Could you check a few things on this model? Use its own coordinates, in mm. Face numbers are marked on the shaded views. A direction names the side the tool comes from. Give positions to 0.01 mm unless a question says otherwise; leave off trailing zeros. Order: outer loops, then holes, each group sorted by start corner. A loop starts at its lowest first (then second) coordinate and runs counter-clockwise, first axis right, second up. Notation, with made-up numbers: M 32.25,77.25 L 48.25,77.25 A24 ccw 48.25,94.25 Z; hole C 44.25,-18.5 d10. An arc over 180 degrees is marked long. Return JSON: item names as keys, results as strings. Group by question number.
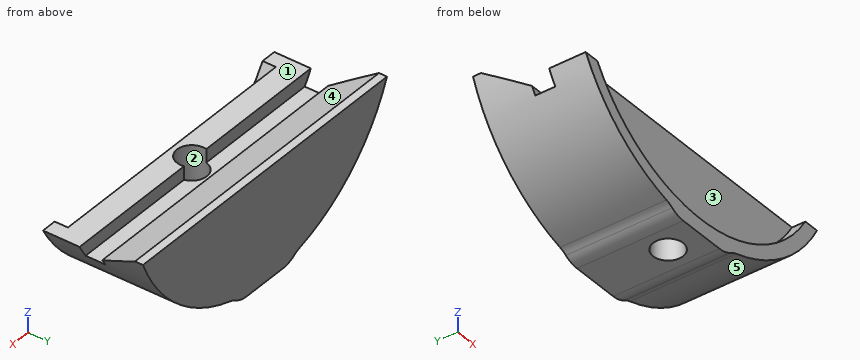
```python
from build123d import *

# Parameters (mm, degrees)
SKETCH_1_R                  = 26
EXTRUDE_1_DEPTH             = 14
CUT_EXTRUDE_1_DEPTH         = 30
HOLE_WIZARD_M32_D           = 3.4
HOLE_WIZARD_M32_CBORE_D     = 6.6
HOLE_WIZARD_M32_CBORE_DEPTH = 3
EXTRUDE_START               = 2
SKETCH_12_R                 = 26
SKETCH_12_R_2               = 24
EXTRUDE_2_DEPTH             = 2
CUT_EXTRUDE_START           = -8
CUT_EXTRUDE_4_DEPTH         = 8
FILLET_2_R                  = 1
SKETCH_18_R                 = 6
CUT_EXTRUDE_5_DEPTH         = 3
CUT_EXTRUDE_START_2         = -10
CUT_EXTRUDE_6_DEPTH         = 10
M4X0_71_D                   = 3.3
M4X0_71_DEPTH               = 11.5
M4X0_71_TIP                 = 0.991420021
SKETCH_20_W                 = 50.531548996
SKETCH_20_H                 = 7
CUT_EXTRUDE_7_DEPTH         = 2
SKETCH_24_W                 = 22.63069338
SKETCH_24_H                 = 1
EXTRUDE_3_DEPTH             = 2
SKETCH_25_W                 = 27.749072331
SKETCH_25_H                 = 11.312162615
CUT_EXTRUDE_8_DEPTH         = 60.799665638
SKETCH_26_W                 = 2
SKETCH_26_H                 = 3
CUT_EXTRUDE_10_DEPTH        = 59.164737265
EXTRUDE_START_2             = -16
EXTRUDE_5_DEPTH             = 16
FILLET_3_R                  = 4
FILLET_4_R                  = 4
HOLE_WIZARD_M41_D           = 4.5


with BuildPart() as part:
    # Эскиз1 → Бобышка-Вытянуть1 (new body)
    with BuildSketch(Plane(origin=(0, 0, 0), x_dir=(1, 0, 0), z_dir=(0, 1, 0))):
        with Locations(Location((0, 0, 0), (0, 0, 270))):
            Circle(SKETCH_1_R)
    extrude(amount=EXTRUDE_1_DEPTH)

    # Эскиз2 → Вырез-Вытянуть1 (cut, symmetric)
    with BuildSketch(Plane(origin=(0, 0, 0), x_dir=(0, 0, -1), z_dir=(1, 0, 0))):
        Polygon((13.654700538, 6), (-13.654700538, 6), (-9.728718708, 12.8), (-9.728718708, 14), (9.728718708, 14), (9.728718708, 12.8), align=None)
    extrude(amount=CUT_EXTRUDE_1_DEPTH, both=True, mode=Mode.SUBTRACT)

    # Цековка для винта с внутренним шестигранником M32 (through all)
    with Locations(Plane(origin=(0, 6, 0), x_dir=(1, 0, 0), z_dir=(0, 1, 0))):
        with Locations((-12.5, 0), (12.5, 0), (-6, 0), (6, 0)):
            CounterBoreHole(HOLE_WIZARD_M32_D / 2, HOLE_WIZARD_M32_CBORE_D / 2, HOLE_WIZARD_M32_CBORE_DEPTH)

    # Эскиз12 → Бобышка-Вытянуть2 (add)
    with BuildSketch(Plane.XZ.offset(EXTRUDE_START)):
        with Locations(Location((0, 0, 0), (0, 0, 270))):
            Circle(SKETCH_12_R)
        with Locations(Location((0, 0, 0), (0, 0, 270))):
            Circle(SKETCH_12_R_2, mode=Mode.SUBTRACT)
    extrude(amount=-EXTRUDE_2_DEPTH)

    # Эскиз17 → Вырез-Вытянуть4 (cut)
    with BuildSketch(Plane(origin=(0, 14, 0), x_dir=(1, 0, 0), z_dir=(0, 1, 0)).offset(CUT_EXTRUDE_START)):
        with BuildLine():
            Line((-24.111242861, -9.728718708), (24.111242861, -9.728718708))
            ThreePointArc((24.111242861, -9.728718708), (0, -26), (-24.111242861, -9.728718708))
        make_face()
    extrude(amount=CUT_EXTRUDE_4_DEPTH, mode=Mode.SUBTRACT)

    # Скругление2
    fillet_2_edges = [part.edges().sort_by_distance(p)[0] for p in [
        (9.25, 4.5, -0.572276157),
        (9.25, 4.5, 0.572276157),
        (-9.25, 4.5, 0.572276157),
        (-9.25, 4.5, -0.572276157),
    ]]
    fillet(fillet_2_edges, radius=FILLET_2_R)

    # Эскиз18 → Вырез-Вытянуть5 (cut)
    with BuildSketch(Plane.XZ):
        Circle(SKETCH_18_R)
    extrude(amount=-CUT_EXTRUDE_5_DEPTH, mode=Mode.SUBTRACT)

    # Эскиз19 → Вырез-Вытянуть6 (cut)
    with BuildSketch(Plane(origin=(0, 6, 0), x_dir=(1, 0, 0), z_dir=(0, 1, 0)).offset(CUT_EXTRUDE_START_2)):
        with BuildLine():
            Line((-22.313739765, -13.345299462), (22.313739765, -13.345299462))
            ThreePointArc((22.313739765, -13.345299462), (0, -26), (-22.313739765, -13.345299462))
        make_face()
    extrude(amount=CUT_EXTRUDE_6_DEPTH, mode=Mode.SUBTRACT)

    # Отверстие обработанное метчиком M4x0.71
    with Locations(Plane.XY.offset(13.345299462)):
        with Locations((0, 3)):
            Hole(M4X0_71_D / 2, depth=M4X0_71_DEPTH)
            with Locations((0, 0, -(M4X0_71_DEPTH + M4X0_71_TIP / 2))):  # 118° drill point
                Cone(0, M4X0_71_D / 2, M4X0_71_TIP, mode=Mode.SUBTRACT)

    # Эскиз20 → Вырез-Вытянуть7 (cut)
    with BuildSketch(Plane.XY.offset(13.345299462)):
        with Locations((0, 1.5)):
            Rectangle(SKETCH_20_W, SKETCH_20_H)
    extrude(amount=-CUT_EXTRUDE_7_DEPTH, mode=Mode.SUBTRACT)

    # Эскиз24 → Бобышка-Вытянуть3 (add)
    with BuildSketch(Plane.XY.offset(11.345299462)):
        with Locations((0, 0.5)):
            Rectangle(SKETCH_24_W, SKETCH_24_H)
    extrude(amount=EXTRUDE_3_DEPTH)

    # Эскиз25 → Вырез-Вытянуть8 (cut, through all)
    with BuildSketch(Plane(origin=(26, 0, 0), x_dir=(0, 0, -1), z_dir=(1, 0, 0))):
        with Locations((-1.469835628, 0.343918692)):
            Rectangle(SKETCH_25_W, SKETCH_25_H)
    extrude(amount=-CUT_EXTRUDE_8_DEPTH, mode=Mode.SUBTRACT)

    # Эскиз26 → Вырез-Вытянуть10 (cut, through all)
    with BuildSketch(Plane(origin=(26, 0, 0), x_dir=(0, 0, -1), z_dir=(1, 0, 0))):
        with Locations((13.404700538, 5)):
            Rectangle(SKETCH_26_W, SKETCH_26_H)
    extrude(amount=-CUT_EXTRUDE_10_DEPTH, mode=Mode.SUBTRACT)

    # Эскиз27 → Бобышка-Вытянуть5 (add)
    with BuildSketch(Plane(origin=(0, 14, 0), x_dir=(1, 0, 0), z_dir=(0, 1, 0)).offset(EXTRUDE_START_2)):
        with BuildLine():
            Line((-5, 26.228718708), (5, 26.228718708))
            Line((5, 26.228718708), (5, 25.514701644))
            ThreePointArc((5, 25.514701644), (0, 26), (-5, 25.514701644))
            Line((-5, 25.514701644), (-5, 26.228718708))
        make_face()
    extrude(amount=EXTRUDE_5_DEPTH)

    # Скругление3
    # the kernel refuses this fillet: 4 mm, written as the material it adds along each edge
    with BuildSketch(Plane(origin=(5, -2, -25.514701644), x_dir=(0.9734574738252592, 0, 0.22886796773193235), z_dir=(0, 1, 0))) as fillet_3_piece_1:
        with BuildLine():
            CenterArc((2.09399194, 3.997202592), FILLET_3_R, 235.642702264, 32.214353504)
            Line((-0.163415634, 0.695065247), (-0.208563786, 0.6290225))
            ThreePointArc((-0.208563786, 0.6290225), (-0.159584415, 0.329223186), (-0.077876598, -0.018309437))
            Line((-0.077876598, -0.018309437), (0.002991417, -0.079944052))
            ThreePointArc((0.002991417, -0.079944052), (0.972210544, -0.061816847), (1.94142967, -0.079944052))
            Line((1.94142967, -0.079944052), (1.944421087, 0))
        make_face()
    extrude(amount=16)
    with BuildSketch(Plane(origin=(-5, -2, -25.514701644), x_dir=(-0.9734574738252595, 0, 0.2288679677319309), z_dir=(0, 1, 0))) as fillet_3_piece_2:
        with BuildLine():
            CenterArc((2.09399194, -3.997202592), FILLET_3_R, 92.142944232, 32.214353504)
            Line((-0.163415634, -0.695065247), (-0.208563786, -0.6290225))
            ThreePointArc((-0.208563786, -0.6290225), (-0.159584415, -0.329223186), (-0.077876598, 0.018309437))
            Line((-0.077876598, 0.018309437), (0.002991417, 0.079944052))
            ThreePointArc((0.002991417, 0.079944052), (0.972210544, 0.061816847), (1.94142967, 0.079944052))
            Line((1.94142967, 0.079944052), (1.944421087, 0))
        make_face()
    extrude(amount=16)

    # Скругление4
    fillet_4_edges = [part.edges().sort_by_distance(p)[0] for p in [
        (5, 6, -26.228718708),
        (-5, 6, -26.228718708),
    ]]
    fillet(fillet_4_edges, radius=FILLET_4_R)

    # Отверстие с зазором M41 (through all)
    with Locations(Plane(origin=(0, 0, -26.228718708), x_dir=(-1, 0, 0), z_dir=(0, 0, -1))):
        with Locations((0, 3)):
            Hole(HOLE_WIZARD_M41_D / 2)


solid = part.part
```
1. I need wall thicknesses on L1, parallel to Y at x = 0, z = -19; L2, parallel to Y at x = -4, z = -22.5; L3, parallel to X at y = 3, z = -16.5. Which ranges of each line are inside material? Lowest first, please. Write a range as from..to.
2. Which directions (+Z, -Z, +X, -X, +Y, -Y) give clear straight access to the entire face, cutting with the end or side of a thin tool? Please do the marked faces 4 and 5.
3. Imagine slicing it at D-D, the plane x = -17. Please give me the cut outline in (y, z), plus the area to 3 significant figures.
4. Imagine slicing it at C-C, the plane z = -20.25. Please give me the cut outline in (x, y).
5. For pin 1 (2 mm diameter, centred on x = -18.5, y = 3.5, fed in from +Z); pin 2 (1.5 mm diameter, centred on x = -8, y = 5.5, fed in from +Z); pin 3 (2 mm diameter, centred on y = 9.5, z = -23.5, fed in from +X); pin 4 (3 mm diameter, centred on x = -17.5, z = -20, fed in from -Y), each with a flat end and sliding along its axis, tell me the tip position at first contact or that it passes through.
6. If we mould it in two halves opening along Y, with no side actions, what happens to the marked faces 1, 2 and 3? For each: pulls with the +Y half, pulls with the -Y half, needs draft (parallel to the pull), parting line crosses it, or undercut.
7. Imagine slicing it at A-A, the plane y = 3. Please give me the cut outline in (x, z), plus the area to 3 significant figures.
8. Imagine slicing it at B-B, the plane x = 0. Please give me the cut outline in (y, z).
Values:
{
 "1": {"L1": "y = 0..0.75, 5.25..14", "L2": "y = 0..14", "L3": "x = -20.09..-2.25, 2.25..20.09"},
 "2": {"face 4": "+Z, +X, -X", "face 5": "-Z, +X, +Y, -Y"},
 "3": {"outline": "M -2,-19.67 L 14,-19.67 L 14,-9.73 L 12.8,-9.73 L 6.5,-13.37 L 6.5,-14.4 L 3.5,-14.4 L 3.5,-12.4 L 0,-12.4 L 0,-16.94 L -2,-16.94 Z", "area": "110 mm²"},
 "4": {"outline": "M -16.31,-2 L -12.88,-2 L -12.88,0 L 12.88,0 L 12.88,-2 L 16.31,-2 L 16.31,14 L -16.31,14 Z; hole C 0,3 d4.5"},
 "5": {"pin 1": "stops at z = -12.4", "pin 2": "stops at z = -14.4", "pin 3": "stops at x = 13.03", "pin 4": "stops at y = -2"},
 "6": {"face 1": "needs draft", "face 2": "undercut", "face 3": "pulls with the -Y half"},
 "7": {"outline": "M -22.85,-12.4 A26 ccw -6.89,-25.07 A4 cw -5.77,-25.58 A4 ccw -3.58,-26.23 L -2.25,-26.23 L -2.25,-12.4 Z; M 2.25,-26.23 L 3.58,-26.23 A4 ccw 5.77,-25.58 A4 cw 6.89,-25.07 A26 ccw 22.85,-12.4 L 2.25,-12.4 Z", "area": "384 mm²"},
 "8": {"outline": "M -2,-26.23 L 0.75,-26.23 L 0.75,-12.4 L 0,-12.4 L 0,-24 L -2,-24 Z; M 5.25,-26.23 L 14,-26.23 L 14,-9.73 L 12.8,-9.73 L 6.5,-13.37 L 6.5,-14.4 L 5.25,-14.4 Z"}
}
